Geometry check sheet. Reference: the model listing, model coordinates, mm. A direction names the side the tool comes from. Coordinates: 2 decimals unless noted, no trailing zeros. Order: outer loops, then holes, each group sorted by start corner. A loop starts at its lowest first (then second) coordinate and runs counter-clockwise, first axis right, second up. Notation, with made-up numbers: M 58,-21 L 91,-21 A24 cw 91,17 Z; hole C -16,47 d5. An arc over 180 degrees is marked long. One line per item, written item: value. Start each with the question number.
1) Draft check along X on faces 1 (the flat face through (12.5, -0.1, -0.5)), 2 (the flat face through (-3, 4, -0.5)), 3 (the flat face through (3, 0, 0)). Enter one of: pulls with the +X half, pulls with the -X half, needs draft (parallel to the pull), parting line crosses it, or undercut.
2) Sectioned sample at B-B, the plane x = 2. Enter the section's corners in (y, z).
3) Thickness scan on L1, parallel to Y at x = -1.5, z = -0.8; L2, parallel to Y at x = -4.25, z = -0.2; L3, parallel to X at y = 1, z = -0.15. Record the ranges inside material, lowest first. Write a range as from..to.
4) Go/stop test with a flat-tipped pin: P1, Ø1.2, axis at x = -4, y = 3, coming from the -Z side. Record where the tip stops, or that it passes through.
5) Access from +Z, -Z, +X, -X, +Y, -Y to the whole of each face (thin tool, end or side, straight path). Record for faces 4 (the flat face through (3, 0, -1)), 5 (the flat face through (2.5, -0.1, -0.6)).
6) Sectioned sample at A-A, the plane y = -2.25. Enter the section's corners in (x, z).
7) Sectioned sample at C-C, the plane z = -0.2. Enter the section's corners in (x, y), then the cut area to 3 significant figures.
```python
from build123d import *

# Parameters (mm, degrees)
F0_W     = 25
F0_H     = 14.999996
F1_DEPTH = 1.000001
F2_W     = 9.99998
F2_H     = 4.99999
F3_DEPTH = 25.4
F4_W     = 9.99998
F4_H     = 9.99998
F5_DEPTH = 0.499999


with BuildPart() as f1:
    # F0 (on Top) → F1 (new body)
    with BuildSketch(Plane.XY):
        Rectangle(F0_W, F0_H)
    extrude(amount=-F1_DEPTH)

    # F2 (on face) → F3 (cut)
    with BuildSketch(Plane.XY):
        with Locations((-2.499995, 0)):
            Rectangle(F2_W, F2_H)
    extrude(amount=-F3_DEPTH, mode=Mode.SUBTRACT)

    # F4 (on face) → F5 (cut)
    with BuildSketch(Plane(origin=(0, 0, -1.000001), x_dir=(1, 0, 0), z_dir=(0, 0, -1))):
        with Locations((-2.499995, 0)):
            Rectangle(F4_W, F4_H)
    extrude(amount=-F5_DEPTH, mode=Mode.SUBTRACT)


solid = f1.part
```
Final values:
1. face 1: pulls with the +X half
1. face 2: undercut
1. face 3: needs draft
2. outline: M -7.5,-1 L -5,-1 L -5,-0.5 L -2.5,-0.5 L -2.5,0 L -7.5,0 Z; M 2.5,-0.5 L 5,-0.5 L 5,-1 L 7.5,-1 L 7.5,0 L 2.5,0 Z
3. L1: y = -7.5..-5, 5..7.5
3. L2: y = -7.5..-2.5, 2.5..7.5
3. L3: x = -12.5..-7.5, 2.5..12.5
4. P1: stops at z = -0.5
5. face 4: -Z, +X, -X, +Y, -Y
5. face 5: -Z
6. outline: M -12.5,-1 L -7.5,-1 L -7.5,0 L -12.5,0 Z; M 2.5,-1 L 12.5,-1 L 12.5,0 L 2.5,0 Z
7. outline: M -12.5,-7.5 L 12.5,-7.5 L 12.5,7.5 L -12.5,7.5 Z; hole M -7.5,-2.5 L 2.5,-2.5 L 2.5,2.5 L -7.5,2.5 Z
7. area: 325 mm^2
